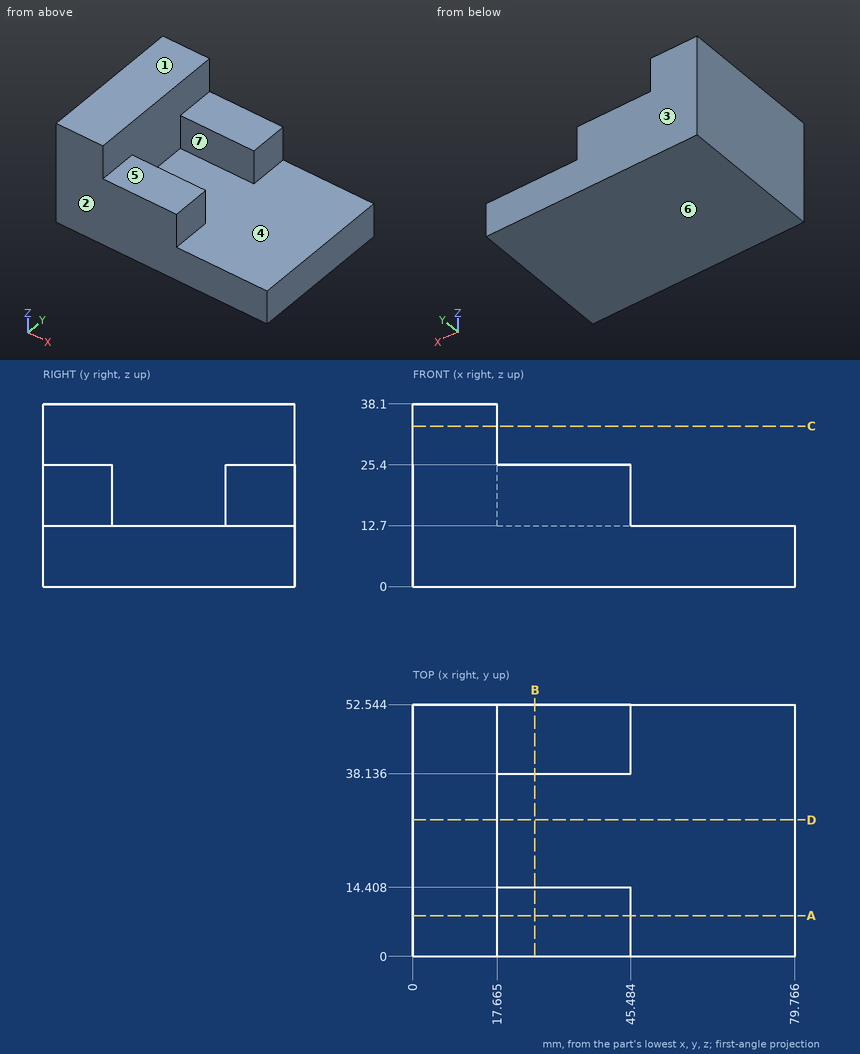
The drawing under review shows one solid part. Ordinate dimensions are in mm from its lowest x, y, z. A direction names the side the tool comes from. Coordinates: 2 decimals unless noted, no trailing zeros. Loops run counter-clockwise (first coordinate to the right, second up) from the corner with the lowest first, then second, coordinate; pieces in that order, holes last. Notation, with made-up numbers: (81, -16.75) -> (131, -16.75) arc R26 cw to (131, 10.25) -> close; hole circle Ø6 at (63.25, 77). An arc over 180 degrees is marked (long way). Answer as a JSON object with one key per item and string values.
Q1. Take a section at B-B on x = 25.5. Give the boundary of the cut face in (y, z) (1 decimal), plus the area to 3 significant figures.
Answer block:
{"outline": "(0, 0) -> (52.5, 0) -> (52.5, 25.4) -> (38.1, 25.4) -> (38.1, 12.7) -> (14.4, 12.7) -> (14.4, 25.4) -> (0, 25.4) -> close", "area": "1,030 mm^2"}
Q2. Take a section at C-C on z = 33.5. Give the boundary of the cut face in (x, y) (1 decimal).
Answer block:
{"outline": "(0, 0) -> (17.7, 0) -> (17.7, 52.5) -> (0, 52.5) -> close"}
Q3. Take a section at D-D on y = 28.5. Give the boundary of the cut face in (x, z) (1 decimal), plus the area to 3 significant figures.
Answer block:
{"outline": "(0, 0) -> (79.8, 0) -> (79.8, 12.7) -> (17.7, 12.7) -> (17.7, 38.1) -> (0, 38.1) -> close", "area": "1,460 mm^2"}
Q4. Tool access review of the marked faces 5, 6 and 7: name each direction out of +Z, -Z, +X, -X, +Y, -Y from which nothing blocks a thin tool from reaching the whole face with its end or side.
Answer block:
{"face 5": "+Z, +X, +Y, -Y", "face 6": "-Z, +X, -X, +Y, -Y", "face 7": "+Z, +X"}
Q5. Clearance check with flat-ended pins moving along their axes: pin 1 Ø4 at (x, y) = (55, 33.5) entering from -Z; pin 2 Ø4 at (x, y) = (36.5, 23.5) entering from +Z; pin 3 Ø11.5 at (x, y) = (29.5, 43) entering from +Z; pin 4 Ø10 at (y, z) = (45, 22) entering from +X. State where each tip first meets the part, or that it passes through.
Answer block:
{"pin 1": "stops at z = 0", "pin 2": "stops at z = 12.7", "pin 3": "stops at z = 25.4", "pin 4": "stops at x = 45.48"}
Q6. The part is to be moulded in two halves that separate along Y. For the marked faces 1, 2, 3 and 4, say which applies: +Y half, -Y half, draft (parallel to the pull), parting line (faces both ways), or undercut.
Answer block:
{"face 1": "draft", "face 2": "-Y half", "face 3": "+Y half", "face 4": "undercut"}
Q7. Take a section at A-A on y = 8.5. Give the boundary of the cut face in (x, z) (1 decimal).
Answer block:
{"outline": "(0, 0) -> (79.8, 0) -> (79.8, 12.7) -> (45.5, 12.7) -> (45.5, 25.4) -> (17.7, 25.4) -> (17.7, 38.1) -> (0, 38.1) -> close"}
Q8. To check wall thickness, follow L1, parallel to Z at x = 34, y = 45.5; L2, parallel to Z at x = 48.5, y = 46; L3, parallel to X at y = 27.5, z = 36 (1 decimal). State the ranges of each line that lie inside material, in increasing order.
Answer block:
{"L1": "z = 0 to 25.4", "L2": "z = 0 to 12.7", "L3": "x = 0 to 17.7"}
